Verification items for the finished model (mm, model axes). A direction names the side the tool comes from. Coordinates: 2 decimals unless noted, no trailing zeros. Order: outer loops, then holes, each group sorted by start corner. A loop starts at its lowest first (then second) coordinate and runs counter-clockwise, first axis right, second up. Notation, with made-up numbers: M 48.5,51.5 L 81.5,51.5 A22 cw 81.5,59.5 Z; hole C 69.5,-22.75 d4. An arc over 180 degrees is marked long. Return JSON: item names as keys, results as strings.
```python
from build123d import *
from build123d.topology import SkipClean

# Parameters (mm, degrees)
SKETCH1_R           = 9.525
SKETCH1_R_2         = 6.604
BOSS_EXTRUDE1_DEPTH = 2.54
BOSS_EXTRUDE2_START = 7.62
SKETCH2_R           = 7.62
SKETCH2_R_2         = 6.604
BOSS_EXTRUDE2_DEPTH = 7.62
BOSS_EXTRUDE3_START = 20.955
SKETCH3_R           = 7.62
SKETCH3_R_2         = 6.096
BOSS_EXTRUDE3_DEPTH = 20.955
SKETCH5_W           = 3.81
SKETCH5_H           = 26.035
CUT_EXTRUDE1_DEPTH  = 37.780699762
SKETCH7_W           = 3.81
SKETCH7_H           = 26.035
CUT_EXTRUDE2_DEPTH  = 37.780699762


with BuildPart() as part:
    # Sketch1 → Boss-Extrude1 (new body)
    with BuildSketch(Plane(origin=(0, 0, 0), x_dir=(1, 0, 0), z_dir=(0, 1, 0))):
        with Locations(Location((0, 0, 0), (0, 0, 270))):
            Circle(SKETCH1_R)
        with Locations(Location((0, 0, 0), (0, 0, 270))):
            Circle(SKETCH1_R_2, mode=Mode.SUBTRACT)
    extrude(amount=BOSS_EXTRUDE1_DEPTH)

    # Sketch2 → Boss-Extrude2 (add)
    with SkipClean():  # the faces are left unmerged after this step: merging them gives an invalid solid
        with BuildSketch(Plane(origin=(0, 0, 0), x_dir=(-1, 0, 0), z_dir=(0, -1, 0)).offset(BOSS_EXTRUDE2_START)):
            with Locations(Location((0, 0, 0), (0, 0, 270))):
                Circle(SKETCH2_R)
            with Locations(Location((0, 0, 0), (0, 0, 90))):
                Circle(SKETCH2_R_2, mode=Mode.SUBTRACT)
        extrude(amount=-BOSS_EXTRUDE2_DEPTH)

    # Sketch3 → Boss-Extrude3 (add)
    with SkipClean():  # the faces are left unmerged after this step: merging them gives an invalid solid
        with BuildSketch(Plane(origin=(0, -7.62, 0), x_dir=(-1, 0, 0), z_dir=(0, -1, 0)).offset(BOSS_EXTRUDE3_START)):
            with Locations(Location((0, 0, 0), (0, 0, 270))):
                Circle(SKETCH3_R)
            with Locations(Location((0, 0, 0), (0, 0, 90))):
                Circle(SKETCH3_R_2, mode=Mode.SUBTRACT)
        extrude(amount=-BOSS_EXTRUDE3_DEPTH)

    # Sketch5 → Cut-Extrude1 (cut, through all)
    with SkipClean():  # the faces are left unmerged after this step: merging them gives an invalid solid
        with BuildSketch(Plane(origin=(0, -28.575, 7.62), x_dir=(1, 0, 0), z_dir=(0, 0, 1))):
            with Locations((0, 15.5575)):
                Rectangle(SKETCH5_W, SKETCH5_H)
        extrude(amount=-CUT_EXTRUDE1_DEPTH, mode=Mode.SUBTRACT)
    add(part.part.scale(1), mode=Mode.REPLACE)  # the faces are merged on a copy

    # Sketch7 → Cut-Extrude2 (cut, through all)
    with BuildSketch(Plane(origin=(7.62, -28.575, 0), x_dir=(0, 0, -1), z_dir=(1, 0, 0))):
        with Locations((0, 15.5575)):
            Rectangle(SKETCH7_W, SKETCH7_H)
    extrude(amount=-CUT_EXTRUDE2_DEPTH, mode=Mode.SUBTRACT)


solid = part.part
```
Q1. Cross-section at B-B, the plane z = 0. Record the boundary of the cut face in (x, y) (3 decimals), and give its area (3 significant figures).
Values:
{"outline": "M -9.525,0 L -6.604,0 L -6.604,2.54 L -9.525,2.54 Z; M -7.62,-28.575 L -6.096,-28.575 L -6.096,-26.035 L -7.62,-26.035 Z; M 6.096,-28.575 L 7.62,-28.575 L 7.62,-26.035 L 6.096,-26.035 Z; M 6.604,0 L 9.525,0 L 9.525,2.54 L 6.604,2.54 Z", "area": "22.6 mm^2"}
Q2. Material ranges on line 1 along Z through (x, y) = (0, 1.45) (3 decimals); line 2 along Y through (x, z) = (-7, 1) (3 decimals), recorded low to high.
Values:
{"line 1": "-9.525 to -6.604, 6.604 to 9.525", "line 2": "-28.575 to -26.035, 0 to 2.54"}
Q3. Go/stop test with flat-tipped pins: pin 1 (1.3 mm diameter, centred on y = -13.5, z = -7, fed in from +X); pin 2 (1.7 mm diameter, centred on x = 6.5, y = -8.5, fed in from -Z); pin 3 (2 mm diameter, centred on x = -4.5, z = -3, fed in from +Y). Record where each tip stops, or that it passes through.
Values:
{"pin 1": "x = 4.21", "pin 2": "z = -5.11", "pin 3": "y = -7.62"}
Q4. Cross-section at C-C, the plane z = 3.5. Record the boundary of the cut face in (x, y) (3 decimals).
Values:
{"outline": "M -8.859,0 L -6.769,0 L -6.769,-28.575 L -4.991,-28.575 L -4.991,-7.62 L -5.6,-7.62 L -5.6,2.54 L -8.859,2.54 Z; M 4.991,-28.575 L 6.769,-28.575 L 6.769,0 L 8.859,0 L 8.859,2.54 L 5.6,2.54 L 5.6,-7.62 L 4.991,-7.62 Z"}
Q5. Draft check along Y on faces 1 (the face through (-5.796, 1.252, -7.559)), 2 (the face through (-7, -13, 1.905)), 3 (the face through (-4.5, -7.62, 4.4)), 4 (the face through (-6, -28.575, 2)). Enter one of: pulls with the +Y half, pulls with the -Y half, needs draft (parallel to the pull), parting line crosses it, or undercut.
Values:
{"face 1": "needs draft", "face 2": "undercut", "face 3": "pulls with the +Y half", "face 4": "pulls with the -Y half"}
Q6. Tool access check on faces 5 (the face through (-2, 2.54, -6.5)), 6 (the face through (1.905, -13, -7)), 7 (the face through (5, -7.62, 4)), 8 (the face through (7, -13, 1.905)), 9 (the face through (-2.289, -14.488, 7.268)). Record the directions out of +Z, -Z, +X, -X, +Y, -Y that give a thin tool (end or side, any length) a straight path to the whole face; none if there is none.
Values:
{"face 5": "+Z, -Z, +X, -X, +Y", "face 6": "+Z, -Z", "face 7": "+Y", "face 8": "+X, -X", "face 9": "-Y"}
Q7. Cross-section at A-A, the plane x = 0. Record the boundary of the cut face in (y, z) (3 decimals), and give its area (3 significant figures).
Values:
{"outline": "M -28.575,-7.62 L -26.035,-7.62 L -26.035,-6.096 L -28.575,-6.096 Z; M -28.575,6.096 L -26.035,6.096 L -26.035,7.62 L -28.575,7.62 Z; M 0,-9.525 L 2.54,-9.525 L 2.54,-6.604 L 0,-6.604 Z; M 0,6.604 L 2.54,6.604 L 2.54,9.525 L 0,9.525 Z", "area": "22.6 mm^2"}
